Drawing for the job (mm, zero at the part's lowest x, y, z). A direction names the side the tool comes from. Round coordinates to 2 decimals unless told otherwise and drop trailing zeros. Write each loop counter-clockwise with the first axis right and the second up, starting at its lowest first coordinate (ties: lowest second). Pieces come first, ordered by that corner, then holes.
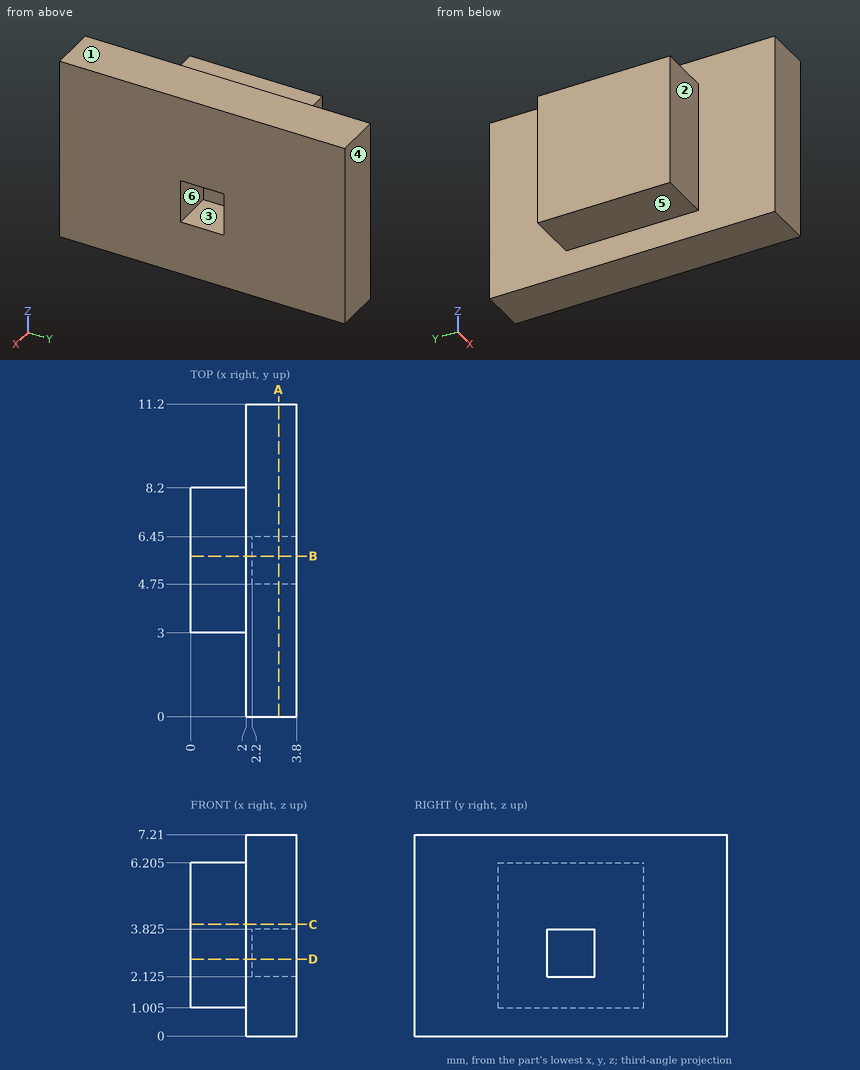
1) Wall check: probe 1 along Z at (x, y) = (3.3, 5) (3 decimals); probe 2 along Y at (x, z) = (2.25, 3); probe 3 along X at (y, z) = (10.5, 5.5). Give the ranges that are in metal, low to high.
2) Pull direction Z, two halves, no side cores. Call the marked faces 4, 5 and 6: released by +Z, released by -Z, zero draft, split by the parting line, or undercut.
3) Cut at A-A on x = 3.15. List the corners of the cut face in (y, z) (3 decimals), and give its area (3 significant figures).
4) Cut at B-B on y = 5.75. List the corners of the cut face in (x, z) (3 decimals).
5) Flat gauge pins, fed straight in: pin 1 Ø0.6 at (x, y) = (1, 7) entering from -Z (3 decimals); pin 2 Ø1.5 at (x, z) = (1, 1) entering from -Y; pin 3 Ø2 at (x, y) = (0.5, 7.5) entering from +Z (3 decimals). Where does each tip first touch, or does it go through?
6) Cut at C-C on z = 4. List the corners of the cut face in (x, y).
7) Cut at D-D on z = 2.75. List the corners of the cut face in (x, y), and give its area (3 significant figures).
8) Which spindle directions (+Z, -Z, +X, -X, +Y, -Y) get a long thin tool onto all of the face, cutting with end or side? Do the marked faces 1, 2 and 3. Say none if no direction does.
Result sheet:
1. probe 1: z = 0 to 2.125, 3.825 to 7.21
1. probe 2: y = 0 to 4.75, 6.45 to 11.2
1. probe 3: x = 2 to 3.8
2. face 4: zero draft
2. face 5: released by -Z
2. face 6: undercut
3. outline: (0, 0) - (11.2, 0) - (11.2, 7.21) - (0, 7.21) - close; hole (4.75, 2.125) - (6.45, 2.125) - (6.45, 3.825) - (4.75, 3.825) - close
3. area: 77.9 mm2
4. outline: (0, 1.005) - (2, 1.005) - (2, 0) - (3.8, 0) - (3.8, 2.125) - (2.2, 2.125) - (2.2, 3.825) - (3.8, 3.825) - (3.8, 7.21) - (2, 7.21) - (2, 6.205) - (0, 6.205) - close
5. pin 1: stops at z = 1.005
5. pin 2: stops at y = 3
5. pin 3: stops at z = 6.205
6. outline: (0, 3) - (2, 3) - (2, 0) - (3.8, 0) - (3.8, 11.2) - (2, 11.2) - (2, 8.2) - (0, 8.2) - close
7. outline: (0, 3) - (2, 3) - (2, 0) - (3.8, 0) - (3.8, 4.75) - (2.2, 4.75) - (2.2, 6.45) - (3.8, 6.45) - (3.8, 11.2) - (2, 11.2) - (2, 8.2) - (0, 8.2) - close
7. area: 27.8 mm2
8. face 1: +Z, +X, -X, +Y, -Y
8. face 2: +Z, -Z, -X, -Y
8. face 3: +X
